from build123d import *

# Parameters (mm, degrees)
F0_W     = 241.3
F0_H     = 38.1
F1_DEPTH = 38.1


with BuildPart() as f1:
    # F0 (on Front) → F1 (new body)
    with BuildSketch(Plane.XZ):
        Polygon((711.2, 0), (711.2, 396.875), (241.3, 396.875), (241.3, 358.775), (673.1, 358.775), (673.1, 0), align=None)
        with Locations((120.65, 377.825)):
            Rectangle(F0_W, F0_H)
        Polygon((711.2, -396.875), (711.2, 0), (673.1, 0), (673.1, -358.775), (241.3, -358.775), (241.3, -396.875), align=None)
        with Locations((-120.65, 377.825)):
            Rectangle(F0_W, F0_H)
        Polygon((-241.3, 358.775), (-241.3, 396.875), (-711.2, 396.875), (-711.2, 0), (-673.1, 0), (-673.1, 358.775), align=None)
        with Locations((120.65, -377.825)):
            Rectangle(F0_W, F0_H)
        with Locations((-120.65, -377.825)):
            Rectangle(F0_W, F0_H)
        Polygon((-673.1, 0), (-711.2, 0), (-711.2, -396.875), (-241.3, -396.875), (-241.3, -358.775), (-673.1, -358.775), align=None)
    extrude(amount=F1_DEPTH)


solid = f1.part
The model under review builds one solid part; all positions refer to its coordinate system, in mm. A direction names the side the tool comes from. Round coordinates to 2 decimals unless told otherwise and drop trailing zeros. Loops run counter-clockwise (first coordinate to the right, second up) from the corner with the lowest first, then second, coordinate; pieces in that order, holes last. Notation, with made-up numbers: (82.5, 2.5) -> (122.5, 2.5) arc R4 ccw to (122.5, 9.5) -> close; hole circle Ø11 at (-19, 41.25). An arc over 180 degrees is marked (long way). Write item = value, one per line. Start each with the question number.
Item 1: To check wall thickness, follow L1, parallel to Z at x = -328, y = -32 (3 decimals); L2, parallel to X at y = -35, z = 319. State the ranges of each line that lie inside material, in increasing order.
Item 2: Take a section at A-A on z = 17. Give the boundary of the cut face in (x, y), plus the area to 3 significant figures.
Item 3: Take a section at B-B on x = -564. Give the boundary of the cut face in (y, z) (3 decimals).
Item 4: For faces 4 (the flat face through (711.2, -19, -6)), 5 (the flat face through (673.1, -19, 5)), list the 3-axis set-ups (+Z, -Z, +X, -X, +Y, -Y) from which the entire face can be reached by the end or side of a thin tool; tool diameter is ignored.
Item 5: Take a section at C-C on y = -8. Give the boundary of the cut face in (x, z) (3 decimals).
Item 6: Mouldability with a two-part tool opening along Z and no side actions: class faces 1 (the flat face through (9, -19, -358.775)), 2 (the flat face through (-56, 0, -380)), 3 (the flat face through (10, -19, 396.875)) as released by +Z, released by -Z, zero draft, split by the parting line, or undercut.
Result:
q1.L1 = -396.875 to -358.775, 358.775 to 396.875
q1.L2 = -711.2 to -673.1, 673.1 to 711.2
q2.outline = (-711.2, -38.1) -> (-673.1, -38.1) -> (-673.1, 0) -> (-711.2, 0) -> close; (673.1, -38.1) -> (711.2, -38.1) -> (711.2, 0) -> (673.1, 0) -> close
q2.area = 2,900 mm²
q3.outline = (-38.1, -396.875) -> (0, -396.875) -> (0, -358.775) -> (-38.1, -358.775) -> close; (-38.1, 358.775) -> (0, 358.775) -> (0, 396.875) -> (-38.1, 396.875) -> close
q4.face_4 = +Z, -Z, +X, +Y, -Y
q4.face_5 = +Y, -Y
q5.outline = (-711.2, -396.875) -> (711.2, -396.875) -> (711.2, 396.875) -> (-711.2, 396.875) -> close; hole (-673.1, -358.775) -> (673.1, -358.775) -> (673.1, 358.775) -> (-673.1, 358.775) -> close
q6.face_1 = undercut
q6.face_2 = zero draft
q6.face_3 = released by +Z
